The model under review builds one solid part; all positions refer to its coordinate system, in mm. Face numbers are marked on the shaded views. Round coordinates to 2 decimals unless told otherwise and drop trailing zeros. Order: outer loops, then holes, each group sorted by start corner. A loop starts at its lowest first (then second) coordinate and runs counter-clockwise, first axis right, second up. Notation, with made-up numbers: M 22,-14.5 L 36,-14.5 A17 cw 36,-4.5 Z; hole C -34,-14.5 d10. An arc over 180 degrees is marked long. Answer as CSV lines item,"result". Start each with the question number.
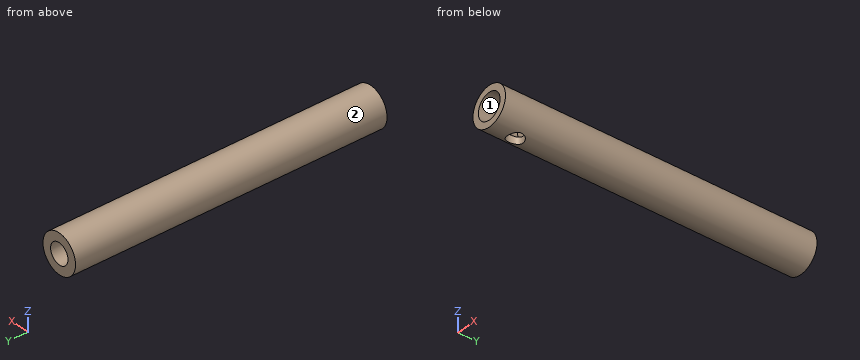
from build123d import *

# Parameters (mm, degrees)
SKETCH1_R           = 7.5
BOSS_EXTRUDE1_DEPTH = 120
SKETCH2_R           = 5
CUT_EXTRUDE1_DEPTH  = 15
SKETCH3_R           = 3
CUT_EXTRUDE4_DEPTH  = 10
SKETCH4_R           = 4
CUT_EXTRUDE5_DEPTH  = 12


with BuildPart() as part:
    # Sketch1 → Boss-Extrude1 (new body)
    with BuildSketch(Plane(origin=(0, 0, 0), x_dir=(1, 0, 0), z_dir=(0, 1, 0))):
        Circle(SKETCH1_R)
    extrude(amount=BOSS_EXTRUDE1_DEPTH)

    # Sketch2 → Cut-Extrude1 (cut)
    with BuildSketch(Plane.XZ):
        Circle(SKETCH2_R)
    extrude(amount=-CUT_EXTRUDE1_DEPTH, mode=Mode.SUBTRACT)

    # Sketch3 → Cut-Extrude4 (cut)
    with BuildSketch(Plane.XY):
        with Locations((0, 10)):
            Circle(SKETCH3_R)
    extrude(amount=-CUT_EXTRUDE4_DEPTH, mode=Mode.SUBTRACT)

    # Sketch4 → Cut-Extrude5 (cut)
    with BuildSketch(Plane(origin=(0, 120, 0), x_dir=(1, 0, 0), z_dir=(0, 1, 0))):
        Circle(SKETCH4_R)
    extrude(amount=-CUT_EXTRUDE5_DEPTH, mode=Mode.SUBTRACT)


solid = part.part
Item 1: For pin 1 (7 mm diameter, centred on x = 0, z = 0, fed in from +Y); pin 2 (1.5 mm diameter, centred on y = 65, z = -4.5, fed in from +X); pin 3 (1.5 mm diameter, centred on y = 33, z = -6, fed in from -X), all flat-tipped, find the tip position at first contact; note any pin that passes through.
Item 2: The part is to be moulded in two halves that separate along Z. For the marked faces 1 and 2, say which applies: +Z half, -Z half, draft (parallel to the pull), parting line (faces both ways), or undercut.
Item 3: Consider section C-C (y = 112.5). State the section outline as (x, z) points.
Item 4: Consider section D-D (y = 61). State the section outline as (x, z) points.
Item 5: Consider section B-B (z = 0). State the section outline as (x, y) points, and give its area (3 significant figures).
Item 6: Consider section A-A (x = 0). State the section outline as (y, z) points, and give its area (3 significant figures).
Item 7: Wall thickness on probe 1 along Y at (x, z) = (0, -5.4); probe 2 along Y at (x, z) = (0.5, 3.25); probe 3 along Z at (x, y) = (0, 5.5): over which ranges is each line inside the solid? List them lowest first. Write a range as [from, to].
Reported:
1,pin 1,"stops at y = 108"
1,pin 2,"stops at x = 6.5"
1,pin 3,"stops at x = -5.36"
2,face 1,"undercut"
2,face 2,"parting line"
3,outline,"C 0,0 d15; hole C 0,0 d8"
4,outline,"C 0,0 d15"
5,outline,"M -7.5,0 L -5,0 L -5,15 L 5,15 L 5,0 L 7.5,0 L 7.5,120 L 4,120 L 4,108 L -4,108 L -4,120 L -7.5,120 Z"
5,area,"1,550 mm²"
6,outline,"M 0,-7.5 L 7,-7.5 L 7,-5 L 0,-5 Z; M 0,5 L 15,5 L 15,-5 L 13,-5 L 13,-7.5 L 120,-7.5 L 120,-4 L 108,-4 L 108,4 L 120,4 L 120,7.5 L 0,7.5 Z"
6,area,"1,540 mm²"
7,probe 1,"y = [0, 7], [13, 120]"
7,probe 2,"y = [15, 108]"
7,probe 3,"z = [-7.5, -5], [5, 7.5]"
